Solid Edge part; units mm, degrees
sketch "Sketch1" plane through (0, 0, 0) normal (0, -1, 0) x (1, 0, 0)
  line L0 (9.8, 12.4) -> (-9.8, 12.4)
  arc A0 (-9.8, 12.4) -> (-12.4, 9.8) centre (-9.8, 9.8) ccw
  line L1 (-12.4, 9.8) -> (-12.4, -9.8)
  arc A1 (-12.4, -9.8) -> (-9.8, -12.4) centre (-9.8, -9.8) ccw
  line L2 (-9.8, -12.4) -> (9.8, -12.4)
  arc A2 (9.8, -12.4) -> (12.4, -9.8) centre (9.8, -9.8) ccw
  line L3 (12.4, -9.8) -> (12.4, 9.8)
  arc A3 (12.4, 9.8) -> (9.8, 12.4) centre (9.8, 9.8) ccw
  arc A4 (-9.8, 15) -> (-15, 9.8) centre (-9.8, 9.8) ccw
  line L4 (-15, 9.8) -> (-15, -9.8)
  arc A5 (-15, -9.8) -> (-9.8, -15) centre (-9.8, -9.8) ccw
  line L5 (-9.8, -15) -> (9.8, -15)
  arc A6 (9.8, -15) -> (15, -9.8) centre (9.8, -9.8) ccw
  line L6 (15, -9.8) -> (15, 9.8)
  arc A7 (15, 9.8) -> (9.8, 15) centre (9.8, 9.8) ccw
  line L7 (9.8, 15) -> (-9.8, 15)
extrude "Protrusion1" add sketch "Sketch1" against normal blind 25.4
For this review, take the finished solid that the model builds, in its own axes (mm). A direction names the side the tool comes from. Round coordinates to 2 decimals unless told otherwise and drop trailing zeros. Write each loop counter-clockwise with the first axis right and the second up, starting at its lowest first coordinate (ties: lowest second). Pieces come first, ordered by that corner, then holes.
1) For line 1 along Z through (x, y) = (-4.25, 18.5); line 2 along X through (y, z) = (7.25, -11), list the stretches that pass through material, from the lowest coordinate up.
Answer below:
line 1: z = -15 to -12.4, 12.4 to 15
line 2: x = -14.86 to -12.11, 12.11 to 14.86
2) Take a section at C-C on z = 4.75. Give the boundary of the cut face in (x, y), then the cut area to 3 significant figures.
Answer below:
outline: (-15, 0) - (-12.4, 0) - (-12.4, 25.4) - (-15, 25.4) - close; (12.4, 0) - (15, 0) - (15, 25.4) - (12.4, 25.4) - close
area: 132 mm2
3) Mouldability with a two-part tool opening along X and no side actions: class faces 1 (the face through (11.659, 12.522, 11.618)), 2 (the face through (0, 13, -15)), 3 (the face through (-13.517, 12.522, -13.436)) as +X half, -X half, draft (parallel to the pull), parting line (faces both ways), or undercut.
Answer below:
face 1: undercut
face 2: draft
face 3: -X half
4) Take a section at B-B on y = 16.5. Give the boundary of the cut face in (x, z).
Answer below:
outline: (-15, -9.8) arc R5.2 ccw to (-9.8, -15) - (9.8, -15) arc R5.2 ccw to (15, -9.8) - (15, 9.8) arc R5.2 ccw to (9.8, 15) - (-9.8, 15) arc R5.2 ccw to (-15, 9.8) - close; hole (-12.4, -9.8) arc R2.6 ccw to (-9.8, -12.4) - (9.8, -12.4) arc R2.6 ccw to (12.4, -9.8) - (12.4, 9.8) arc R2.6 ccw to (9.8, 12.4) - (-9.8, 12.4) arc R2.6 ccw to (-12.4, 9.8) - close
5) Take a section at A-A on x = 8. Give the boundary of the cut face in (y, z).
Answer below:
outline: (0, -15) - (25.4, -15) - (25.4, -12.4) - (0, -12.4) - close; (0, 12.4) - (25.4, 12.4) - (25.4, 15) - (0, 15) - close
6) Machinability: for faces 4 (the face through (12.4, 13, 0)), 5 (the face through (13.436, 12.522, -13.517)), which of the approach directions +Z, -Z, +X, -X, +Y, -Y give a long, thin tool a straight path to every point of the face, cutting with its end or side? Answer none if there is none.
Answer below:
face 4: +Y, -Y
face 5: -Z, +X, +Y, -Y
7) Take a section at D-D on z = 13. Give the boundary of the cut face in (x, y).
Answer below:
outline: (-13.9, 0) - (13.9, 0) - (13.9, 25.4) - (-13.9, 25.4) - close
